```python
from build123d import *

# Parameters (mm, degrees)
F0_W            = 600
F0_H            = 600
F1_DEPTH        = 10
F3_DEPTH        = 10.001
F3_COPIES_COUNT = 4
F5_R            = 25


# Not quite as in the source:
# - a pattern or mirror of a feature is missing from the dataset's text; its kind, count and spacing are read off the source's solid


with BuildPart() as f1:
    # F0 (on Top) → F1 (new body)
    with BuildSketch(Plane.XY):
        Rectangle(F0_W, F0_H)
    extrude(amount=F1_DEPTH)

    # F2 (on Top) → F3 (cut, through all)
    with BuildSketch(Plane.XY):
        with BuildLine():
            Line((-50, 235), (50, 235))
            ThreePointArc((50, 235), (75, 260), (50, 285))
            Line((50, 285), (-50, 285))
            ThreePointArc((-50, 285), (-75, 260), (-50, 235))
        make_face()
    f3 = extrude(amount=F3_DEPTH, mode=Mode.SUBTRACT)

    # F3_copies: F3 ×4 about axis
    f3_copies_axis = Axis((0, 0, 0), (0, 0, 1))
    for i in range(1, F3_COPIES_COUNT):
        add(f3.rotate(f3_copies_axis, i * 360 / F3_COPIES_COUNT), mode=Mode.SUBTRACT)

    # F5
    f5_edges = [f1.edges().sort_by_distance(p)[0] for p in [
        (-300, -300, 5),
        (-300, 300, 5),
        (300, 300, 5),
        (300, -300, 5),
    ]]
    fillet(f5_edges, radius=F5_R)


solid = f1.part
```
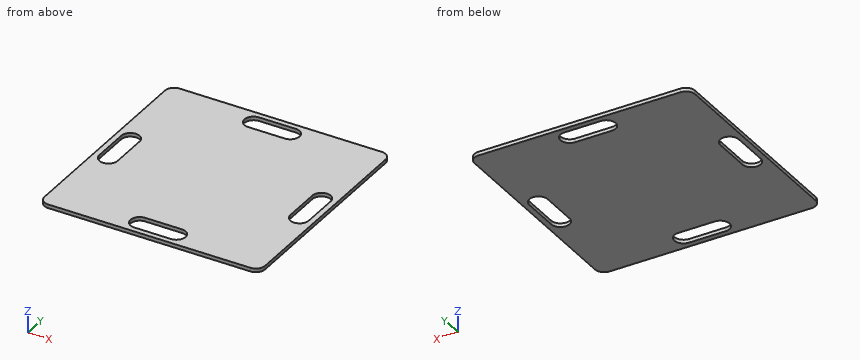
The listing builds one solid part. Answer for the finished solid, in the listing's coordinates (mm). Round coordinates to 2 decimals unless told otherwise and drop trailing zeros. Write each loop counter-clockwise with the first axis right and the second up, starting at its lowest first coordinate (ties: lowest second). Pieces come first, ordered by that corner, then holes. Notation, with made-up numbers: (-22, 19) -> (-11, 19) arc R32 cw to (-11, 50) -> close; hole circle Ø1 at (-18, 6). An arc over 180 degrees is marked (long way). Answer as a JSON object with one key per item and string values. Group by question number.
Q1. Section D-D (z = 4) is taken. Write down the section's boundary in (x, y), plus the area to 3 significant figures.
Q2. Straight lines are drawn through the part: line 1 along X through (y, z) = (-18, 3.5); line 2 along X through (y, z) = (59, 5); line 3 along X through (y, z) = (261, 1). For each, find the intervals that lie inside material, in ascending order.
Q3. Section C-C (y = -10.5) is taken. Write down the section's boundary in (x, z).
Q4. Section A-A (y = -260) is taken. Write down the section's boundary in (x, z), plus the area to 3 significant figures.
Check values:
{
 "1": {"outline": "(-300, -275) arc R25 ccw to (-275, -300) -> (275, -300) arc R25 ccw to (300, -275) -> (300, 275) arc R25 ccw to (275, 300) -> (-275, 300) arc R25 ccw to (-300, 275) -> close; hole (-285, -50) arc R25 ccw to (-235, -50) -> (-235, 50) arc R25 ccw to (-285, 50) -> close; hole (-50, -285) -> (50, -285) arc R25 ccw to (50, -235) -> (-50, -235) arc R25 ccw to start; hole (-50, 235) -> (50, 235) arc R25 ccw to (50, 285) -> (-50, 285) arc R25 ccw to start; hole (235, -50) arc R25 ccw to (285, -50) -> (285, 50) arc R25 ccw to (235, 50) -> close", "area": "332,000 mm^2"},
 "2": {"line 1": "-300 to -285, -235 to 235, 285 to 300", "line 2": "-300 to -283.32, -236.68 to 236.68, 283.32 to 300", "line 3": "-300 to -74.98, 74.98 to 300"},
 "3": {"outline": "(-300, 0) -> (-285, 0) -> (-285, 10) -> (-300, 10) -> close; (-235, 0) -> (235, 0) -> (235, 10) -> (-235, 10) -> close; (285, 0) -> (300, 0) -> (300, 10) -> (285, 10) -> close"},
 "4": {"outline": "(-300, 0) -> (-75, 0) -> (-75, 10) -> (-300, 10) -> close; (75, 0) -> (300, 0) -> (300, 10) -> (75, 10) -> close", "area": "4,500 mm^2"}
}
